For this review, take the finished solid that the model builds, in its own axes (mm). Face numbers are marked on the shaded views. A direction names the side the tool comes from. Round coordinates to 2 decimals unless told otherwise and drop trailing zeros. Loops run counter-clockwise (first coordinate to the right, second up) from the corner with the lowest first, then second, coordinate; pieces in that order, holes last. Notation, with made-up numbers: (64.5, -2.75) -> (76.5, -2.75) arc R23 ccw to (76.5, 19.25) -> close; hole circle Ø5 at (4.5, -28.5). An arc over 180 degrees is marked (long way). Use one line per item in the form item = value. Start each with the question number.
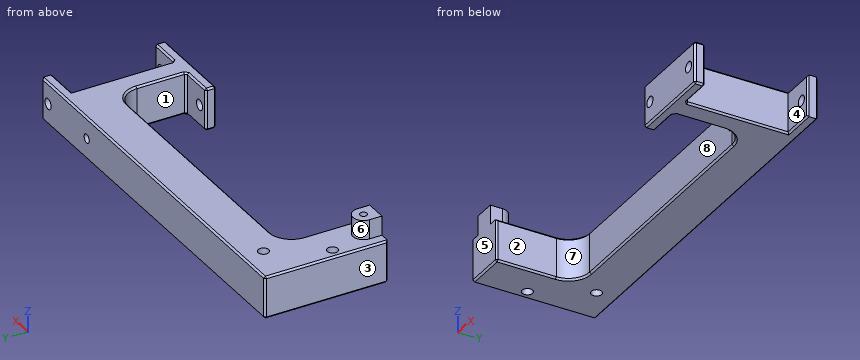
from build123d import *

# Parameters (mm, degrees)
SKETCH1_R                    = 1.5
BOSS_EXTRUDE1_DEPTH          = 6
BOSS_EXTRUDE2_DEPTH          = 5.5
M2_5X0_45_TAPPED_HOLE1_D     = 2.05
M2_5X0_45_TAPPED_HOLE1_DEPTH = 6.234117865
M2_5X0_45_TAPPED_HOLE1_TIP   = 0.615882135
CUT_EXTRUDE1_REACH           = 116.658
SKETCH6_R                    = 1.5
CUT_EXTRUDE2_REACH           = 117.531
SKETCH7_R                    = 1.5
M3X0_5_TAPPED_HOLE1_D        = 2.5
M3X0_5_TAPPED_HOLE1_DEPTH    = 14.5
M3X0_5_TAPPED_HOLE1_TIP      = 0.751075774
CHAMFER1_SIZE                = 0.5


with BuildPart() as part:
    # Sketch1 → Boss-Extrude1 (new, symmetric)
    with BuildSketch(Plane.XY):
        with BuildLine():
            Line((0, 0), (0, 35))
            Line((0, 35), (109.5, 35))
            Line((109.5, 35), (109.5, 32))
            Line((109.5, 32), (100, 32))
            Line((100, 32), (100, 3))
            Line((100, 3), (109.5, 3))
            Line((109.5, 3), (109.5, 0))
            Line((109.5, 0), (84.5, 0))
            Line((84.5, 0), (84.5, 3))
            Line((84.5, 3), (94, 3))
            Line((94, 3), (94, 17))
            ThreePointArc((94, 17), (92.242640687, 21.242640687), (88, 23))
            Line((88, 23), (18, 23))
            ThreePointArc((18, 23), (13.757359313, 21.242640687), (12, 17))
            Line((12, 17), (12, 0))
            Line((12, 0), (0, 0))
        make_face()
        with Locations((11, 29)):
            Circle(SKETCH1_R, mode=Mode.SUBTRACT)
        with Locations((3, 14)):
            Circle(SKETCH1_R, mode=Mode.SUBTRACT)
    extrude(amount=BOSS_EXTRUDE1_DEPTH, both=True)

    # Sketch2 → Boss-Extrude2 (add)
    with BuildSketch(Plane.XY.offset(6)):
        with BuildLine():
            Line((3, 3.5), (3, 0))
            Line((3, 0), (9, 0))
            Line((9, 0), (9, 3.5))
            ThreePointArc((9, 3.5), (6, 6.5), (3, 3.5))
        make_face()
    extrude(amount=BOSS_EXTRUDE2_DEPTH)

    # M2.5x0.45 Tapped Hole1
    with Locations(Plane.XY.offset(11.5)):
        with Locations((6, 3.5)):
            Hole(M2_5X0_45_TAPPED_HOLE1_D / 2, depth=M2_5X0_45_TAPPED_HOLE1_DEPTH)
            with Locations((0, 0, -(M2_5X0_45_TAPPED_HOLE1_DEPTH + M2_5X0_45_TAPPED_HOLE1_TIP / 2))):  # 118° drill point
                Cone(0, M2_5X0_45_TAPPED_HOLE1_D / 2, M2_5X0_45_TAPPED_HOLE1_TIP, mode=Mode.SUBTRACT)

    # Sketch6 → Cut-Extrude1 (cut, up to next)
    with BuildSketch(Plane(origin=(0, 3, 0), x_dir=(1, 0, 0), z_dir=(0, 1, 0)), mode=Mode.PRIVATE) as cut_extrude1_sk1:
        with Locations(Location((87.5, 0, 0), (0, 0, 180))):
            Circle(SKETCH6_R)
    cut_extrude1_tool1 = extrude(cut_extrude1_sk1.sketch, amount=-CUT_EXTRUDE1_REACH, mode=Mode.PRIVATE) & part.part
    # Sketch6 → Cut-Extrude1 (cut, up to next)
    with BuildSketch(Plane(origin=(0, 3, 0), x_dir=(1, 0, 0), z_dir=(0, 1, 0)), mode=Mode.PRIVATE) as cut_extrude1_sk2:
        with Locations(Location((106.5, 0, 0), (0, 0, 180))):
            Circle(SKETCH6_R)
    cut_extrude1_tool2 = extrude(cut_extrude1_sk2.sketch, amount=-CUT_EXTRUDE1_REACH, mode=Mode.PRIVATE) & part.part
    add(cut_extrude1_tool1.solids().sort_by_distance((87.5, 3, 0))[0], mode=Mode.SUBTRACT)
    add(cut_extrude1_tool2.solids().sort_by_distance((106.5, 3, 0))[0], mode=Mode.SUBTRACT)

    # Sketch7 → Cut-Extrude2 (cut, up to next)
    with BuildSketch(Plane(origin=(0, 35, 0), x_dir=(1, 0, 0), z_dir=(0, 1, 0)), mode=Mode.PRIVATE) as cut_extrude2_sk1:
        with Locations(Location((106.5, 0, 0), (0, 0, 180))):
            Circle(SKETCH7_R)
    cut_extrude2_tool1 = extrude(cut_extrude2_sk1.sketch, amount=-CUT_EXTRUDE2_REACH, mode=Mode.PRIVATE) & part.part
    add(cut_extrude2_tool1.solids().sort_by_distance((106.5, 35, 0))[0], mode=Mode.SUBTRACT)

    # M3x0.5 Tapped Hole1
    with Locations(Plane(origin=(0, 35, 0), x_dir=(1, 0, 0), z_dir=(0, 1, 0))):
        with Locations((87.5, 0)):
            Hole(M3X0_5_TAPPED_HOLE1_D / 2, depth=M3X0_5_TAPPED_HOLE1_DEPTH)
            with Locations((0, 0, -(M3X0_5_TAPPED_HOLE1_DEPTH + M3X0_5_TAPPED_HOLE1_TIP / 2))):  # 118° drill point
                Cone(0, M3X0_5_TAPPED_HOLE1_D / 2, M3X0_5_TAPPED_HOLE1_TIP, mode=Mode.SUBTRACT)

    # Chamfer1
    chamfer1_edges = [part.edges().sort_by_distance(p)[0] for p in [
        (12, 8.5, -6),
        (12, 8.5, 6),
        (13.757359313, 21.242640687, -6),
        (13.757359313, 21.242640687, 6),
        (53, 23, -6),
        (53, 23, 6),
        (92.242640687, 21.242640687, -6),
        (92.242640687, 21.242640687, 6),
        (97, 0, 6),
        (109.5, 0, 0),
        (84.5, 0, 0),
        (94, 3, 0),
        (94, 10, -6),
        (89.25, 3, -6),
        (84.5, 1.5, 6),
        (94, 10, 6),
        (89.25, 3, 6),
        (84.5, 3, 0),
        (84.5, 1.5, -6),
        (97, 0, -6),
        (100, 3, 0),
        (109.5, 1.5, 6),
        (109.5, 1.5, -6),
        (104.75, 32, -6),
        (109.5, 32, 0),
        (104.75, 32, 6),
        (100, 17.5, -6),
        (104.75, 3, -6),
        (109.5, 3, 0),
        (104.75, 3, 6),
        (100, 17.5, 6),
        (0, 17.5, -6),
        (12, 0, 0),
        (6, 0, -6),
        (0, 35, 0),
        (0, 0, 0),
        (54.75, 35, -6),
        (109.5, 35, 0),
        (54.75, 35, 6),
        (0, 17.5, 6),
    ]]
    chamfer(chamfer1_edges, length=CHAMFER1_SIZE)


solid = part.part
Item 1: For P1, Ø1.5, axis at y = 7.5, z = -2, coming from the +X side; P2, Ø9, axis at x = 61.5, z = -2.5, coming from the -Y side; P3, Ø3.5, axis at x = 3, y = 14, coming from the +Z side, all flat-tipped, find the tip position at first contact; note any pin that passes through.
Item 2: Take a section at A-A on z = 3. Give the number of separate pieces and of enclosed holes in the cut face, plus the area to 3 significant figures.
Item 3: Draft analysis for pull direction X (two halves, no side actions). For the marked faces 5, 6, 7 and 8, state which applies: +X half, -X half, draft (parallel to the pull), parting line (faces both ways), or undercut.
Item 4: Machinability: for the marked faces 1, 2, 3 and 4, which of the approach directions +Z, -Z, +X, -X, +Y, -Y give a long, thin tool a straight path to every point of the face, cutting with its end or side? Answer none if there is none.
Item 5: Take a section at C-C on x = 35. Give the boundary of the cut face in (y, z), plus the area to 4 significant figures.
Item 6: Take a section at D-D on z = 8. Give the boundary of the cut face in (x, y) (3 decimals), plus the area to 3 significant figures.
Item 7: Wall thickness on line 1 (Y direction, x = 11, z = 1.5); line 2 (X direction, y = 26.5, z = -2.25); line 3 (Y direction, x = 3, z = 3.75): over which ranges is each line inside the solid? List them lowest first.
Item 8: Take a section at B-B on y = 14. Give the boundary of the cut face in (x, z).
Results:
q1.P1 = 100
q1.P2 = 23
q1.P3 = 6
q2.separate_pieces = 1
q2.enclosed_holes = 2
q2.area = 1,700 mm2
q3.face_5 = draft
q3.face_6 = parting line
q3.face_7 = undercut
q3.face_8 = undercut
q4.face_1 = +Z, -Z
q4.face_2 = +Z, -Z, -Y
q4.face_3 = +Z, -Z, -X, +Y, -Y
q4.face_4 = +Z, -Z, +X
q5.outline = (23, -5.5) -> (23.5, -6) -> (34.5, -6) -> (35, -5.5) -> (35, 5.5) -> (34.5, 6) -> (23.5, 6) -> (23, 5.5) -> close
q5.area = 143.5 mm2
q6.outline = (3, 0) -> (9, 0) -> (9, 3.5) arc R3 ccw to (3, 3.5) -> close; hole circle Ø2.05 at (6, 3.5)
q6.area = 31.8 mm2
q7.line_1 = 0 to 27.5, 30.5 to 35
q7.line_2 = 0 to 100
q7.line_3 = 0 to 12.5, 15.5 to 35
q8.outline = (0, -5.5) -> (0.5, -6) -> (1.5, -6) -> (1.5, 6) -> (0.5, 6) -> (0, 5.5) -> close; (4.5, -6) -> (11.5, -6) -> (12, -5.5) -> (12, 5.5) -> (11.5, 6) -> (4.5, 6) -> close; (94, -5.5) -> (94.5, -6) -> (99.5, -6) -> (100, -5.5) -> (100, 5.5) -> (99.5, 6) -> (94.5, 6) -> (94, 5.5) -> close
